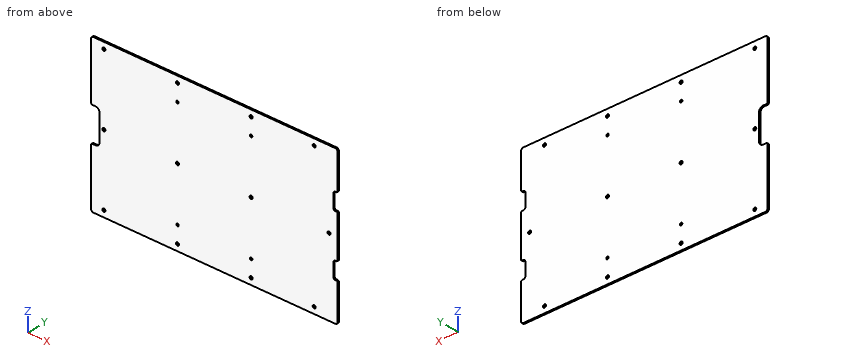
```python
from build123d import *

# Parameters (mm, degrees)
SKETCH1_R           = 2.2479
SKETCH1_R_2         = 1.8288
BOSS_EXTRUDE1_DEPTH = 2.286
CUT_EXTRUDE1_DEPTH  = 217.750866886
FILLET1_R           = 1.5875


with BuildPart() as part:
    # Sketch1 → Boss-Extrude1 (new body)
    with BuildSketch(Plane(origin=(0, 0, 0), x_dir=(1, 0, 0), z_dir=(0, 1, 0))):
        with BuildLine():
            Line((-180.975, 114.3), (180.975, 114.3))
            ThreePointArc((180.975, 114.3), (183.22006403, 113.37006403), (184.15, 111.125))
            Line((184.15, 111.125), (184.15, -111.125))
            ThreePointArc((184.15, -111.125), (183.22006403, -113.37006403), (180.975, -114.3))
            Line((180.975, -114.3), (-180.975, -114.3))
            ThreePointArc((-180.975, -114.3), (-183.22006403, -113.37006403), (-184.15, -111.125))
            Line((-184.15, -111.125), (-184.15, 111.125))
            ThreePointArc((-184.15, 111.125), (-183.22006403, 113.37006403), (-180.975, 114.3))
        make_face()
        with Locations(Location((-165.1, 104.775, 0), (0, 0, 270))):
            Circle(SKETCH1_R, mode=Mode.SUBTRACT)
        with Locations(Location((-55.033333333, 104.775, 0), (0, 0, 270))):
            Circle(SKETCH1_R, mode=Mode.SUBTRACT)
        with Locations(Location((55.033333333, 104.775, 0), (0, 0, 270))):
            Circle(SKETCH1_R, mode=Mode.SUBTRACT)
        with Locations(Location((55.033333333, -104.775, 0), (0, 0, 270))):
            Circle(SKETCH1_R, mode=Mode.SUBTRACT)
        with Locations(Location((-55.033333333, -104.775, 0), (0, 0, 270))):
            Circle(SKETCH1_R, mode=Mode.SUBTRACT)
        with Locations(Location((-165.1, -104.775, 0), (0, 0, 270))):
            Circle(SKETCH1_R, mode=Mode.SUBTRACT)
        with Locations(Location((-55.033333333, 0, 0), (0, 0, 270))):
            Circle(SKETCH1_R, mode=Mode.SUBTRACT)
        with Locations(Location((55.033333333, 0, 0), (0, 0, 270))):
            Circle(SKETCH1_R, mode=Mode.SUBTRACT)
        with Locations(Location((149.225, -104.775, 0), (0, 0, 270))):
            Circle(SKETCH1_R, mode=Mode.SUBTRACT)
        with Locations(Location((149.225, 104.775, 0), (0, 0, 270))):
            Circle(SKETCH1_R, mode=Mode.SUBTRACT)
        with Locations(Location((55.0291, -80.01, 0), (0, 0, 270))):
            Circle(SKETCH1_R_2, mode=Mode.SUBTRACT)
        with Locations(Location((-55.0291, -80.01, 0), (0, 0, 270))):
            Circle(SKETCH1_R_2, mode=Mode.SUBTRACT)
        with Locations(Location((-55.0291, 80.01, 0), (0, 0, 270))):
            Circle(SKETCH1_R_2, mode=Mode.SUBTRACT)
        with Locations(Location((55.0291, 80.01, 0), (0, 0, 270))):
            Circle(SKETCH1_R_2, mode=Mode.SUBTRACT)
        with Locations(Location((171.45, 0, 0), (0, 0, 270))):
            Circle(SKETCH1_R, mode=Mode.SUBTRACT)
        with Locations(Location((-165.1, 0, 0), (0, 0, 270))):
            Circle(SKETCH1_R, mode=Mode.SUBTRACT)
    extrude(amount=BOSS_EXTRUDE1_DEPTH)

    # Sketch2 → Cut-Extrude1 (cut, through all)
    with BuildSketch(Plane.XZ):
        with BuildLine():
            Line((184.15, 57.658), (180.975, 57.658))
            ThreePointArc((180.975, 57.658), (178.72993597, 56.72806403), (177.8, 54.483))
            Line((177.8, 54.483), (177.8, 35.433))
            ThreePointArc((177.8, 35.433), (178.72993597, 33.18793597), (180.975, 32.258))
            Line((180.975, 32.258), (184.15, 32.258))
            Line((184.15, 32.258), (184.15, 57.658))
        make_face()
        with BuildLine():
            Line((184.15, -32.258), (180.975, -32.258))
            ThreePointArc((180.975, -32.258), (178.72993597, -33.18793597), (177.8, -35.433))
            Line((177.8, -35.433), (177.8, -54.483))
            ThreePointArc((177.8, -54.483), (178.72993597, -56.72806403), (180.975, -57.658))
            Line((180.975, -57.658), (184.15, -57.658))
            Line((184.15, -57.658), (184.15, -32.258))
        make_face()
        with BuildLine():
            Line((-184.15, 25.4), (-177.8, 25.4))
            ThreePointArc((-177.8, 25.4), (-173.309871939, 23.540128061), (-171.45, 19.05))
            Line((-171.45, 19.05), (-171.45, -19.05))
            ThreePointArc((-171.45, -19.05), (-173.309871939, -23.540128061), (-177.8, -25.4))
            Line((-177.8, -25.4), (-184.15, -25.4))
            Line((-184.15, -25.4), (-184.15, 25.4))
        make_face()
    extrude(amount=-CUT_EXTRUDE1_DEPTH, mode=Mode.SUBTRACT)

    # Fillet1
    fillet1_edges = [part.edges().sort_by_distance(p)[0] for p in [
        (184.15, 1.143, 57.658),
        (184.15, 1.143, 32.258),
        (184.15, 1.143, -32.258),
        (184.15, 1.143, -57.658),
        (-184.15, 1.143, -25.4),
        (-184.15, 1.143, 25.4),
    ]]
    fillet(fillet1_edges, radius=FILLET1_R)


solid = part.part
```
Part model, mm, in its own coordinate system. Give positions to 0.01 mm unless a question says otherwise; leave off trailing zeros. Order: outer loops, then holes, each group sorted by start corner. A loop starts at its lowest first (then second) coordinate and runs counter-clockwise, first axis right, second up. Notation, with made-up numbers: (-16, -22) - (12, -22) arc R22 cw to (12, 12) - close; hole circle Ø2 at (6.25, 88). An arc over 180 degrees is marked (long way). Use one line per item in the form item = value.
Item 1: Slice it at A-A on z = 47.5. Give the cut face in (x, y), and give its area (3 significant figures).
Solution:
outline = (-184.15, 0) - (177.8, 0) - (177.8, 2.29) - (-184.15, 2.29) - close
area = 827 mm2
Item 2: Pin check, flat tips, straight feed: pin 1 Ø1.3 at (x, y) = (182, 1.5) entering from +Z; pin 2 Ø0.8 at (x, y) = (181.5, 1) entering from -Z. Stop position of each tip, or through.
Solution:
pin_1 = 114.28
pin_2 = -114.3
Item 3: Probe probe 1 along X at (y, z) = (0.7, 0); probe 2 along X at (y, z) = (1.4, -79); probe 3 along X at (y, z) = (0.2, -10.5). List the from-to ranges inside material, lowest first. Write a range as from..to.
Solution:
probe_1 = -171.45..-167.35, -162.85..-57.28, -52.79..52.79, 57.28..169.2, 173.7..184.15
probe_2 = -184.15..-56.55, -53.5..53.5, 56.55..184.15
probe_3 = -171.45..184.15
